Here's how the part is built. I have some questions about the finished solid (model axes, mm). Face numbers are marked on the shaded views. A direction names the side the tool comes from. Coordinates: 2 decimals unless noted, no trailing zeros. Write each loop counter-clockwise with the first axis right and the second up, starting at its lowest first coordinate (ties: lowest second). Pieces come first, ordered by that corner, then holes.
Item 1: If we section it at A-A (y = 0): Please give me the cut outline in (x, z), then the cut area to 3 significant figures.
Item 2: I'm going to push flat-ended pins straight in: pin 1 Ø8 at (x, y) = (0, 0) entering from -Z; pin 2 Ø0.6 at (y, z) = (7.5, -2) entering from -X; pin 3 Ø1.8 at (x, y) = (-6.5, 6) entering from +Z. Where does each tip first touch, or does it pass through?
Item 3: If we section it at D-D (y = -6): Please give me the cut outline in (x, z).
Item 4: If we section it at C-C (z = -2.25): Please give me the cut outline in (x, y).
Item 5: If I drill on line 1 (Y direction, x = 6, z = -6.15); line 2 (X direction, y = -2, z = -7.5); line 3 (X direction, y = -7, z = -2.5), over which ranges is the centre line in solid material (lowest first)?
Item 6: We'd pull the mould along X, two halves only. Please class the marked faces 6, 7 and 8: +X half, -X half, draft (parallel to the pull), parting line (faces both ways), or undercut.
Item 7: For the marked faces 1, 2, 3, 4 and 5, which set-ups out of +Z, -Z, +X, -X, +Y, -Y let a thin tool reach every point of the face, with its end or its side?
Item 8: If we section it at B-B (x = 6.5): Please give me the cut outline in (y, z).
Autodesk Inventor part; units mm, degrees
ref_plane "YZ Plane" through (0, 0, 0) normal (1, 0, 0) x (0, 1, 0)
ref_plane "XZ Plane" through (0, 0, 0) normal (0, 1, 0) x (-1, 0, 0)
ref_plane "XY Plane" through (0, 0, 0) normal (0, 0, 1) x (1, 0, 0)
sketch "Boceto1" plane through (0, 0, 0) normal (0, 0, 1) x (1, 0, 0)
  line L0 (-7.5, -7.5) -> (7.5, -7.5)
  line L1 (7.5, -7.5) -> (7.5, 7.5)
  line L2 (7.5, 7.5) -> (-7.5, 7.5)
  line L3 (-7.5, 7.5) -> (-7.5, -7.5)
  line L4 (-7.5, -7.5) -> (7.5, 7.5) construction
  line L5 (7.5, -7.5) -> (-7.5, 7.5) construction
  dimension "d2" = 15
extrude "Extrusión1" add sketch "Boceto1" against normal blind 8
sketch "Boceto2" plane through (0, 0, -8) normal (0, 0, -1) x (-1, 0, 0)
  circle A0 centre (-6, 6) radius 0.75
  line L0 (6, -6) -> (-6, -6) construction
  line L1 (-6, -6) -> (-6, 6) construction
  line L2 (-6, 6) -> (6, 6) construction
  line L3 (6, 6) -> (6, -6) construction
  line L4 (6, -6) -> (-6, 6) construction
  line L5 (-6, -6) -> (6, 6) construction
  circle A1 centre (6, 6) radius 0.75
  circle A2 centre (6, -6) radius 0.75
  circle A3 centre (-6, -6) radius 0.75
  point P0 (0, 0)
  dimension "d5" = 12
  dimension "d6" = 1.5
extrude "Extrusión2" cut sketch "Boceto2" against normal up to surface (8 mm away)
sketch "Boceto3" plane through (0, 0, 0) normal (0, 0, 1) x (1, 0, 0)
  line L0 (7.5, 7.5) -> (-7.5, 7.5)
  line L1 (-7.5, 7.5) -> (-4, 7.5)
  line L2 (-4, 7.5) -> (-4, 4)
  line L3 (-4, 4) -> (-7.5, 4)
  line L4 (-7.5, 4) -> (-7.5, 7.5)
  line L5 (-7.5, -7.5) -> (-7.5, -4)
  line L6 (-7.5, -4) -> (-4, -4)
  line L7 (-4, -4) -> (-4, -7.5)
  line L8 (-4, -7.5) -> (-7.5, -7.5)
  line L9 (7.5, -7.5) -> (4, -7.5)
  line L10 (4, -7.5) -> (4, -4)
  line L11 (4, -4) -> (7.5, -4)
  line L12 (7.5, -4) -> (7.5, -7.5)
  line L13 (7.5, 7.5) -> (7.5, 4)
  line L14 (7.5, 4) -> (4, 4)
  line L15 (4, 4) -> (4, 7.5)
  line L16 (4, 7.5) -> (7.5, 7.5)
  point P0 (0, 0)
  point P1 (0, 0)
  point P2 (0, 0)
  point P3 (0, 0)
  dimension "d9" = 3.5
  dimension "d12" = 360
extrude "Extrusión3" cut sketch "Boceto3" against normal blind 5
fillet "Empalme1" radius 3 4 edges at (-4, 4, -2.5) (4, 4, -2.5) (4, -4, -2.5) (-4, -4, -2.5)
sketch "Boceto4" plane through (0, 0, -8) normal (0, 0, -1) x (-1, 0, 0)
  line L0 (0, 5.7735) -> (5, 2.8868)
  line L1 (5, 2.8868) -> (5, -2.8868)
  line L2 (5, -2.8868) -> (0, -5.7735)
  line L3 (0, -5.7735) -> (-5, -2.8868)
  line L4 (-5, -2.8868) -> (-5, 2.8868)
  line L5 (-5, 2.8868) -> (0, 5.7735)
  point P0 (0, 0)
  point P1 (0, 0)
  dimension "d17" = 10
extrude "Extrusión4" cut sketch "Boceto4" against normal blind 5
sketch "Boceto5" plane through (0, 0, 0) normal (0, 0, 1) x (1, 0, 0)
  circle A0 centre (0, 0) radius 3
  dimension "d20" = 6
extrude "Extrusión5" cut sketch "Boceto5" against normal up to surface (8 mm away)
properties part number "sujecion_cable"
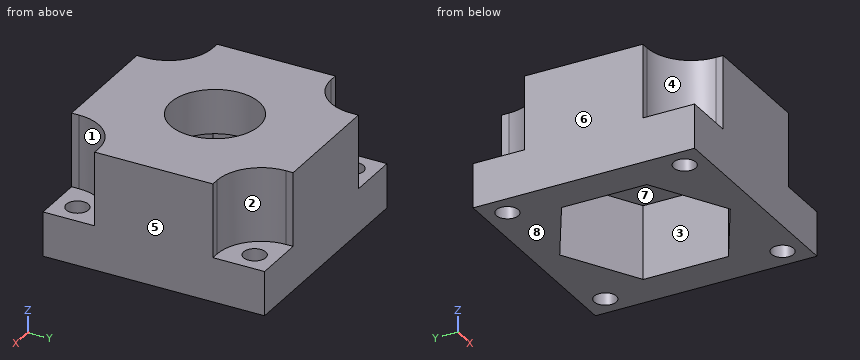
Answer list:
1. outline: (-7.5, -8) - (-5, -8) - (-5, -3) - (-3, -3) - (-3, 0) - (-7.5, 0) - close; (3, -3) - (5, -3) - (5, -8) - (7.5, -8) - (7.5, 0) - (3, 0) - close
1. area: 52.0 mm2
2. pin 1: stops at z = -3
2. pin 2: stops at x = -4
2. pin 3: stops at z = -5
3. outline: (-7.5, -8) - (-6.75, -8) - (-6.75, -5) - (-7.5, -5) - close; (-5.25, -8) - (5.25, -8) - (5.25, -5) - (4.17, -5) - (4.17, 0) - (-4.17, 0) - (-4.17, -5) - (-5.25, -5) - close; (6.75, -8) - (7.5, -8) - (7.5, -5) - (6.75, -5) - close
4. outline: (-7.5, -4) - (-7, -4) arc R3 cw to (-4, -7) - (-4, -7.5) - (4, -7.5) - (4, -7) arc R3 cw to (7, -4) - (7.5, -4) - (7.5, 4) - (7, 4) arc R3 cw to (4, 7) - (4, 7.5) - (-4, 7.5) - (-4, 7) arc R3 cw to (-7, 4) - (-7.5, 4) - close; hole circle Ø6 at (0, 0)
5. line 1: y = -7.5 to -6.75, -5.25 to 5.25, 6.75 to 7.5
5. line 2: x = -7.5 to -5, 5 to 7.5
5. line 3: x = -4 to 4
6. face 6: -X half
6. face 7: undercut
6. face 8: draft
7. face 1: +Z, +X, -Y
7. face 2: +Z, +X, +Y
7. face 3: -Z
7. face 4: +Z, -X, -Y
7. face 5: +Z, -Z, +X, +Y, -Y
8. outline: (-7.5, -8) - (-6.56, -8) - (-6.56, -5) - (-7.5, -5) - close; (-5.44, -8) - (5.44, -8) - (5.44, -5) - (4.04, -5) - (4.04, 0) - (-4.04, 0) - (-4.04, -5) - (-5.44, -5) - close; (6.56, -8) - (7.5, -8) - (7.5, -5) - (6.56, -5) - close
